Check sheet for the modelled part. Datum: model origin and axes. Units: mm. A direction names the side the tool comes from. Coordinates: 2 decimals unless noted, no trailing zeros. Loops run counter-clockwise (first coordinate to the right, second up) from the corner with the lowest first, then second, coordinate; pieces in that order, holes last. Notation, with made-up numbers: (70.5, -15) - (82.5, -15) arc R27 ccw to (82.5, 3) - close; hole circle Ø8 at (43, 30). An arc over 180 degrees is marked (long way). Use a Markdown table: item, result. Add a question column.
1) Go/stop test with flat-tipped pins: P1, Ø2, axis at x = 3, y = -3, coming from the +Z side; P2, Ø1, axis at y = 6, z = 15, coming from the -X side; P3, Ø3, axis at x = 3, y = -2.5, coming from the +Z side; P4, Ø12, axis at x = 81, y = -7.5, coming from the +Z side. Record where each tip stops, or that it passes through.
2) Sectioned sample at C-C, the plane z = 0. Enter the section's corners in (x, y), then the cut area to 3 significant figures.
3) Tool access check on faces 4 (the flat face through (6, 10, 0)), 5 (the flat face through (4, -2, -9.5)), 6 (the flat face through (10, -3, -9)), 7 (the flat face through (10, 3, -12)). Record the directions out of +Z, -Z, +X, -X, +Y, -Y that give a thin tool (end or side, any length) a straight path to the whole face; none if there is none.
4) Draft check along Z on faces 1 (the flat face through (10, -4, -10)), 2 (the flat face through (92.664, -7.089, 33.471)), 3 (the flat face through (4, -2, 9.5)). Enter one of: pulls with the +Z half, pulls with the -Z half, needs draft (parallel to the pull), parting line crosses it, or undercut.
5) Sectioned sample at D-D, the plane x = 39. Enter the section's corners in (y, z).
6) Thickness scan on line 1 (Z direction, x = 5.25, y = 0); line 2 (Z direction, x = 12, y = 4.5); line 3 (X direction, y = 5, z = 19.5). Record the ranges inside material, lowest first.
7) Sectioned sample at A-A, the plane x = 16. State how many separate pieces and enclosed holes the cut face has, then the cut area to 3 significant figures.
Autodesk Inventor part; units mm, degrees
ref_plane "YZ Plane" through (0, 0, 0) normal (1, 0, 0) x (0, 1, 0)
ref_plane "XZ Plane" through (0, 0, 0) normal (0, 1, 0) x (-1, 0, 0)
ref_plane "XY Plane" through (0, 0, 0) normal (0, 0, 1) x (1, 0, 0)
sketch "Sketch1" plane through (0, 0, 0) normal (1, 0, 0) x (0, 1, 0)
  arc A0 (-2, -7.746) -> (-2, 7.746) centre (0, 0) ccw
  line L0 (0, 0) -> (-2, 0)
  line L1 (-2, 7.746) -> (-2, 9)
  line L2 (-2, 9) -> (-4, 9)
  line L3 (-4, 9) -> (-4, 12)
  line L4 (-4, 12) -> (11, 12)
  line L5 (-2, 0) -> (-2, -9)
  line L6 (-2, -9) -> (-4, -9)
  line L7 (-4, -9) -> (-4, -12)
  line L8 (-4, -12) -> (11, -12)
  line L9 (11, -12) -> (11, 12)
  line L10 (11, 12) -> (6, 20.6603)
  line L11 (11, 12) -> (21, 12) construction
  line L12 (6, 20.6603) -> (-2.6603, 15.6603)
  line L13 (-2.6603, 15.6603) -> (-0.547, 12)
  dimension "d0" = 16
  dimension "d1" = 2
  dimension "d2" = 9
  dimension "d3" = 2
  dimension "d4" = 3
  dimension "d5" = 15
  dimension "d6" = 9
  dimension "d7" = 3
  dimension "d8" = 10
  dimension "d9" = 120
  dimension "d10" = 10
extrude "Extrusion1" add sketch "Sketch1" along normal blind 20
ref_plane "Work Plane1" through (20, 8, 0) normal (0, 0, -1) x (-1, 0, 0)
ref_plane "Work Plane2" through (0, 0, 12) normal (0, 1, 0) x (1, 0, 0)
sketch "Sketch3" plane through (0, 0, 12) normal (0, 1, 0) x (1, 0, 0)
  line L0 (0, 21) -> (20, 21)
  line L1 (10, 21) -> (10, 22.5)
  line L2 (10, 22.5) -> (14, 22.5)
  line L3 (14, 22.5) -> (14, 21.5)
  line L4 (14, 21.5) -> (18, 21.5)
  line L5 (18, 21.5) -> (18, 23.5)
  line L6 (18, 23.5) -> (14, 23.5)
  line L7 (14, 23.5) -> (14, 22.5)
  line L8 (10, 22.5) -> (6, 22.5)
  line L9 (6, 22.5) -> (6, 23.5)
  line L10 (6, 23.5) -> (2, 23.5)
  line L11 (2, 23.5) -> (2, 21.5)
  line L12 (2, 21.5) -> (6, 21.5)
  line L13 (6, 22.5) -> (6, 21.5)
  line L14 (0, 3) -> (20, 3)
  line L15 (20, 21) -> (20, 3)
  line L16 (20, 20) -> (20, 4)
  line L17 (20, 12) -> (6.2446, 12)
  line L18 (0, 3) -> (20, 3)
  line L19 (10, 3) -> (10, 1.5)
  line L20 (10, 1.5) -> (14, 1.5)
  line L21 (14, 1.5) -> (14, 2.5)
  line L22 (14, 2.5) -> (18, 2.5)
  line L23 (18, 2.5) -> (18, 0.5)
  line L24 (18, 0.5) -> (14, 0.5)
  line L25 (14, 0.5) -> (14, 1.5)
  line L26 (10, 1.5) -> (6, 1.5)
  line L27 (6, 1.5) -> (6, 0.5)
  line L28 (6, 0.5) -> (2, 0.5)
  line L29 (2, 0.5) -> (2, 2.5)
  line L30 (2, 2.5) -> (6, 2.5)
  line L31 (6, 1.5) -> (6, 2.5)
  point P0 (0, 12)
  point P1 (20, 4.254)
  point P2 (20, 19.746)
  dimension "d25" = 1.5
  dimension "d26" = 4
  dimension "d27" = 1
  dimension "d28" = 4
  dimension "d29" = 2
  dimension "d30" = 4
  dimension "d31" = 1
  dimension "d32" = 4
  dimension "d33" = 2
revolve "Revolution1" cut sketch "Sketch3" angle 180 about axis through (20, 0, 0) along (1, 0, 0) contours L13 L12 L11 L10 L9 | L7 L6 L5 L4 L3
extrude "Extrusion3" cut sketch "Sketch3" against normal blind 20
sketch "Sketch5" plane through (0, 6, 20.6603) normal (0, 0.866, 0.5) x (1, 0, 0)
  line L0 (0, 10) -> (0, 0)
  line L1 (0, 0) -> (20, 0)
  line L2 (0, 0) -> (20, 0)
  arc A0 (93.2847, -16.3126) -> (20, 0) centre (20, -172.7725) ccw
  arc A1 (92.0249, -19.0024) -> (20, -2.9702) centre (20, -172.7725) ccw
  line L3 (20, -2.9702) -> (0, -2.9702)
  line L4 (0, 0) -> (0, -2.9702)
  line L5 (93.2847, -16.3126) -> (92.0249, -19.0024)
  point P0 (0, 14.8923)
extrude "Extrusion4" add sketch "Sketch5" against normal up to surface (10 mm away)
equation "\"BendRadius\" = Thickness"
equation "\"BendReliefWidth\" = Thickness"
equation "\"BendReliefDepth\" = 0.5 * Thickness"
equation "\"CornerReliefSize\" = 4 * Thickness"
equation "\"MinimumRemnant\" = 2 * Thickness"
equation "\"TransitionRadius\" = BendRadius"
equation "\"JacobiRadiusSize\" = BendRadius"
equation "\"GapSize\" = Thickness"
properties part number "abrazadera_leds"
Solved:
| question | item | result |
|---|---|---|
| 1 | P1 | stops at z = 19.47 |
| 1 | P2 | stops at x = 0 |
| 1 | P3 | stops at z = 20.05 |
| 1 | P4 | stops at z = 33.82 |
| 2 | outline | (0, 8) - (20, 8) - (20, 11) - (18, 11) - (18, 9.5) - (14, 9.5) - (14, 11) - (6, 11) - (6, 9.5) - (2, 9.5) - (2, 11) - (0, 11) - close |
| 2 | area | 48.0 mm2 |
| 3 | face 4 | none |
| 3 | face 5 | -Y |
| 3 | face 6 | +X, -X, -Y |
| 3 | face 7 | -Z, +X, -X, +Y, -Y |
| 4 | face 1 | needs draft |
| 4 | face 2 | pulls with the +Z half |
| 4 | face 3 | undercut |
| 5 | outline | (-4.68, 19.16) - (-3.18, 16.57) - (5.48, 21.57) - (3.98, 24.16) - close |
| 6 | line 1 | z = -12 to -11.5, -9.5 to -8, 8 to 9.5, 11.5 to 20.63 |
| 6 | line 2 | z = -12 to -6.61, 6.61 to 23.22 |
| 6 | line 3 | x = 0 to 20 |
| 7 | separate pieces | 3 |
| 7 | enclosed holes | 0 |
| 7 | area | 213 mm2 |
